Here's how the part is built. I have some questions about the finished solid (model axes, mm). Face numbers are marked on the shaded views. Round coordinates to 2 decimals unless told otherwise and drop trailing zeros. Write each loop counter-clockwise with the first axis right and the second up, starting at its lowest first coordinate (ties: lowest second). Pieces come first, ordered by that corner, then holes. Notation, with made-up numbers: (55.5, -11.5) -> (114.5, -11.5) arc R21 ccw to (114.5, 21.5) -> close; hole circle Ø5 at (5.5, 3.5). An arc over 180 degrees is marked (long way). Put each result on its own line as item: value. Start each with the question number.
1) If I drill on line 1 along Z through (x, y) = (-15, -3.5); line 2 along X through (y, z) = (-8, 6.5); line 3 along X through (y, z) = (-2.75, 7.75), over which ranges is the centre line in solid material (lowest first)? Write a range as [from, to].
2) I want a section at A-A, the plane z = 5. List the corners of the cut face in (x, y) for me, then the cut area to 3 significant figures.
3) I want a section at D-D, the plane x = 15.5. List the corners of the cut face in (y, z) for me.
4) Will these pins go through, and if not, where does the flat tip stop? P1, Ø3, axis at x = -3.5, y = -8, coming from the -Z side; P2, Ø6, axis at x = 4, z = 4.5, coming from the +Y side.
5) We'd pull the mould along X, two halves only. Please class the marked faces 1, 2 and 3: released by +X, released by -X, zero draft, split by the parting line, or undercut.
6) I want a section at C-C, the plane y = -5.5. List the corners of the cut face in (x, z) for me.
7) I want a section at B-B, the plane x = -16. List the corners of the cut face in (y, z) for me, then the cut area to 3 significant figures.
from build123d import *

# Parameters (mm, degrees)
BOSS_EXTRUDE1_DEPTH = 10
FILLET1_R           = 2
SKETCH4_R           = 2.6
CUT_EXTRUDE2_DEPTH  = 27.381811917


with BuildPart() as part:
    # Sketch1 → Boss-Extrude1 (new body)
    with BuildSketch(Plane.XY):
        with BuildLine():
            Line((10, 0), (20, 0))
            Line((20, 0), (20, -14))
            Line((20, -14), (-20, -14))
            Line((-20, -14), (-20, 0))
            Line((-20, 0), (-10, 0))
            ThreePointArc((-10, 0), (0, -10), (10, 0))
        make_face()
    extrude(amount=BOSS_EXTRUDE1_DEPTH)

    # Fillet1
    fillet1_edges = [part.edges().sort_by_distance(p)[0] for p in [
        (-20, -7, 10),
        (20, -7, 10),
        (20, -7, 0),
        (-20, -7, 0),
    ]]
    fillet(fillet1_edges, radius=FILLET1_R)

    # Sketch4 → Cut-Extrude2 (cut, through all)
    with BuildSketch(Plane(origin=(0, 0, 0), x_dir=(1, 0, 0), z_dir=(0, 1, 0))):
        with Locations(Location((-15, -5, 0), (0, 0, 180))):
            Circle(SKETCH4_R)
        with Locations(Location((15, -5, 0), (0, 0, 180))):
            Circle(SKETCH4_R)
    extrude(amount=-CUT_EXTRUDE2_DEPTH, mode=Mode.SUBTRACT)


solid = part.part
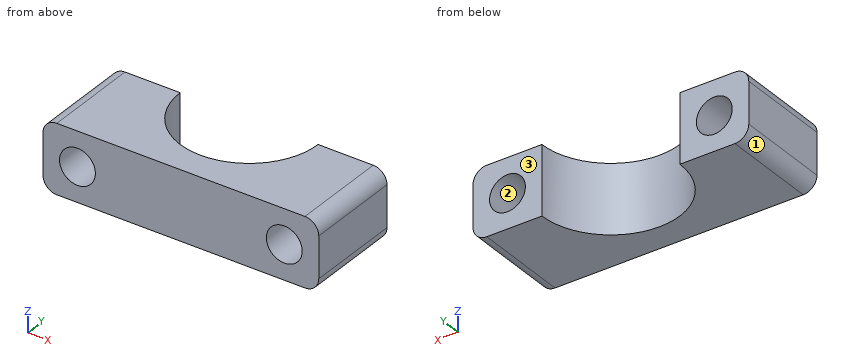
Findings:
1. line 1: z = [0, 2.4], [7.6, 10]
1. line 2: x = [-20, -17.12], [-12.88, -6], [6, 12.88], [17.12, 20]
1. line 3: x = [-20, -9.61], [9.61, 20]
2. outline: (-20, -14) -> (-17.6, -14) -> (-17.6, 0) -> (-20, 0) -> close; (-12.4, -14) -> (12.4, -14) -> (12.4, 0) -> (10, 0) arc R10 cw to (-10, 0) -> (-12.4, 0) -> close; (17.6, -14) -> (20, -14) -> (20, 0) -> (17.6, 0) -> close
2. area: 257 mm2
3. outline: (-14, 0) -> (0, 0) -> (0, 2.45) -> (-14, 2.45) -> close; (-14, 7.55) -> (0, 7.55) -> (0, 10) -> (-14, 10) -> close
4. P1: stops at z = 0
4. P2: stops at y = -7.14
5. face 1: released by -X
5. face 2: undercut
5. face 3: zero draft
6. outline: (-20, 2) arc R2 ccw to (-18, 0) -> (-8.35, 0) -> (-8.35, 10) -> (-18, 10) arc R2 ccw to (-20, 8) -> close; (8.35, 0) -> (18, 0) arc R2 ccw to (20, 2) -> (20, 8) arc R2 ccw to (18, 10) -> (8.35, 10) -> close; hole circle Ø5.2 at (-15, 5); hole circle Ø5.2 at (15, 5)
7. outline: (-14, 0) -> (0, 0) -> (0, 2.6) -> (-14, 2.6) -> close; (-14, 7.4) -> (0, 7.4) -> (0, 10) -> (-14, 10) -> close
7. area: 72.8 mm2
